from build123d import *

# Parameters (mm, degrees)
SKETCH2_R                = 22.225
BOSS_EXTRUDE1_DEPTH      = 152.4
SKETCH3_R                = 28.575
BOSS_EXTRUDE2_DEPTH      = 38.1
BOSS_EXTRUDE2_DEPTH_BACK = 38.1
SKETCH4_R                = 19.05
CUT_EXTRUDE1_DEPTH       = 98.298
FILLET1_R                = 6.35


with BuildPart() as part:
    # Sketch2 → Boss-Extrude1 (new body)
    with BuildSketch(Plane.XY):
        Circle(SKETCH2_R)
    extrude(amount=BOSS_EXTRUDE1_DEPTH)

    # Sketch3 → Boss-Extrude2 (add, two sides)
    with BuildSketch(Plane(origin=(0, 0, 0), x_dir=(1, 0, 0), z_dir=(0, 1, 0))) as boss_extrude2_sk:
        Circle(SKETCH3_R)
    extrude(amount=BOSS_EXTRUDE2_DEPTH)
    extrude(boss_extrude2_sk.sketch, amount=-BOSS_EXTRUDE2_DEPTH_BACK)

    # Sketch4 → Cut-Extrude1 (cut)
    with BuildSketch(Plane(origin=(0, 38.1, 0), x_dir=(1, 0, 0), z_dir=(0, 1, 0))):
        Circle(SKETCH4_R)
    extrude(amount=-CUT_EXTRUDE1_DEPTH, mode=Mode.SUBTRACT)

    # Fillet1
    fillet1_edges = [part.edges().sort_by_distance(p)[0] for p in [
        (-28.575, -38.1, 0),
        (-28.575, 38.1, 0),
    ]]
    fillet(fillet1_edges, radius=FILLET1_R)


solid = part.part
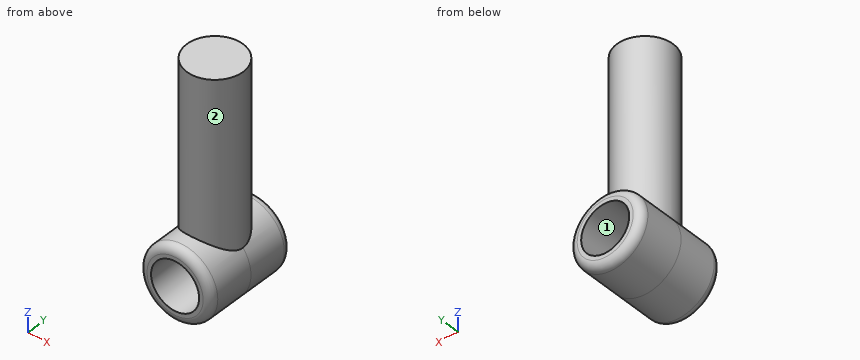
Read the model definition and answer for the solid it produces. Units are mm, in the model's axes. Face numbers are marked on the shaded views. A direction names the side the tool comes from. Coordinates: 2 decimals unless noted, no trailing zeros. Loops run counter-clockwise (first coordinate to the right, second up) from the corner with the lowest first, then second, coordinate; pieces in that order, holes last. Notation, with made-up numbers: (34.5, -2) -> (62.5, -2) arc R29 ccw to (62.5, 28) -> close; hole circle Ø9 at (-17.75, -30). An arc over 180 degrees is marked (long way). Write item = value, one per line. Start each with the question number.
1) For the marked faces 1 and 2, determine the directions among +Z, -Z, +X, -X, +Y, -Y from which every point of the face is accessible in a straight line to the end or side of a thin tool.
2) The part is cut by section C-C, the plane y = -19.5. Determine the outline of the cut face in (x, z) (3 decimals).
3) The part is cut by section B-B, the plane z = 0. Determine the outline of the cut face in (x, y) (3 decimals), plus the area to 3 significant figures.
4) Given P1, Ø12, axis at y = 25, z = 56, coming from the +X side; P2, Ø8, axis at y = -14, z = 28.5, coming from the -X side; P3, Ø5, axis at x = 7, z = 51, coming from the -Y side, each flat-ended and moving along its own axis, determine where each tip first touches the part or whether it passes through.
5) The part is cut by section A-A, the plane x = 0. Determine the outline of the cut face in (y, z) (3 decimals), plus the area to 3 significant figures.
6) Find the intervals of material crossed by L1, parallel to X at y = 22, z = 0 (3 decimals); L2, parallel to Z at x = 0, y = 15 (3 decimals); L3, parallel to Z at x = 9, y = -6.5, in increasing order. Write a range as from..to.
7) The part is cut by section D-D, the plane z = 41.5. Determine the outline of the cut face in (x, y) (3 decimals).
Result:
q1.face_1 = +Y, -Y
q1.face_2 = +Z
q2.outline = (-10.663, 26.511) arc R28.575 ccw (long way) to (10.663, 26.511) -> (10.663, 152.4) -> (-10.663, 152.4) -> close; hole circle Ø38.1 at (0, 0)
q3.outline = (-28.575, -31.75) arc R6.35 ccw to (-22.225, -38.1) -> (-19.05, -38.1) -> (-19.05, 38.1) -> (-22.225, 38.1) arc R6.35 ccw to (-28.575, 31.75) -> close; (19.05, -38.1) -> (22.225, -38.1) arc R6.35 ccw to (28.575, -31.75) -> (28.575, 31.75) arc R6.35 ccw to (22.225, 38.1) -> (19.05, 38.1) -> close
q3.area = 1,420 mm²
q4.P1 = 11.53
q4.P2 = -19.85
q4.P3 = -21.76
q5.outline = (-38.1, -22.225) arc R6.35 ccw to (-31.75, -28.575) -> (31.75, -28.575) arc R6.35 ccw to (38.1, -22.225) -> (38.1, -19.05) -> (-38.1, -19.05) -> close; (-38.1, 19.05) -> (38.1, 19.05) -> (38.1, 22.225) arc R6.35 ccw to (31.75, 28.575) -> (22.225, 28.575) -> (22.225, 152.4) -> (-22.225, 152.4) -> (-22.225, 28.575) -> (-31.75, 28.575) arc R6.35 ccw to (-38.1, 22.225) -> close
q5.area = 6,920 mm²
q6.L1 = -28.575..-19.05, 19.05..28.575
q6.L2 = -28.575..-19.05, 19.05..152.4
q6.L3 = -27.12..-16.79, 16.79..152.4
q7.outline = circle Ø44.45 at (0, 0)
